```python
from build123d import *

# Parameters (mm, degrees)
CYLINDER003003_R     = 2.85
CYLINDER003003_DEPTH = 10
BOX001001004_W       = 1
BOX001001004_H       = 0.2
BOX001001004_DEPTH   = 5.1
CYLINDER002007_R     = 3.4
CYLINDER002007_DEPTH = 8.5
BOX001001005_W       = 1
BOX001001005_H       = 0.2
BOX001001005_DEPTH   = 5.1
CYLINDER004009_R     = 5
CYLINDER004009_DEPTH = 4
CHAMFER008_SIZE      = 0.5
CYLINDER001006_R     = 4
CYLINDER001006_DEPTH = 4.6
CUT003009_ROLL_ANGLE = -90


with BuildPart() as hole001:
    # Cylinder003003 → Cylinder003003 (new body)
    with BuildSketch(Plane.XY):
        Circle(CYLINDER003003_R)
    extrude(amount=CYLINDER003003_DEPTH)


with BuildPart() as contact003:
    # Box001001004 → Box001001004 (new body)
    with BuildSketch(Plane(origin=(-0.5, 2.5, -13), x_dir=(1, 0, 0), z_dir=(0, 0, 1))):
        with Locations((0.5, 0.1)):
            Rectangle(BOX001001004_W, BOX001001004_H)
    extrude(amount=BOX001001004_DEPTH)


with BuildPart() as cylinder002007:
    # Cylinder002007 → Cylinder002007 (new body)
    with BuildSketch(Plane.XY.offset(-8)):
        Circle(CYLINDER002007_R)
    extrude(amount=CYLINDER002007_DEPTH)


with BuildPart() as contact004:
    # Box001001005 → Box001001005 (new body)
    with BuildSketch(Plane(origin=(-0.5, -2.5, -13), x_dir=(1, 0, 0), z_dir=(0, 0, 1))):
        with Locations((0.5, 0.1)):
            Rectangle(BOX001001005_W, BOX001001005_H)
    extrude(amount=BOX001001005_DEPTH)


with BuildPart() as chamfer008:
    # Cylinder004009 → Cylinder004009 (new body)
    with BuildSketch(Plane.XY):
        Circle(CYLINDER004009_R)
    extrude(amount=CYLINDER004009_DEPTH)

    # Chamfer008
    chamfer008_edges = [chamfer008.edges().sort_by_distance(p)[0] for p in [
        (-5, 0, 4),
    ]]
    chamfer(chamfer008_edges, length=CHAMFER008_SIZE)


with BuildPart() as powerconnector:
    # Cylinder001006 → Cylinder001006 (new body)
    with BuildSketch(Plane.XY.offset(-4.5)):
        Circle(CYLINDER001006_R)
    extrude(amount=CYLINDER001006_DEPTH)

    # Fusion005: union contact003, Cylinder002007, contact004, Chamfer008
    add(contact003.part)
    add(cylinder002007.part)
    add(contact004.part)
    add(chamfer008.part)

    # Cut003009: cut hole001
    add(hole001.part, mode=Mode.SUBTRACT)


with BuildPart() as powerconnector_1:
    # Cut003009 roll: moved
    add(powerconnector.part.rotate(Axis((0, 0, 0), (1, 0, 0)), CUT003009_ROLL_ANGLE))


with BuildPart() as powerconnector_2:
    # Cut003009 placement: moved
    add(powerconnector_1.part.moved(Location((-0.7, 30, 39.2))))


solid = powerconnector_2.part
```
Work out the finished part from the listing and answer in its coordinate system (mm). A direction names the side the tool comes from. Give positions to 0.01 mm unless a question says otherwise; leave off trailing zeros. Write each loop counter-clockwise with the first axis right and the second up, starting at its lowest first coordinate (ties: lowest second). Pieces come first, ordered by that corner, then holes.
(1) Flat-ended cylindrical pins translate along their axes: pin 1 Ø3 at (x, z) = (-0.5, 40.5) entering from +Y; pin 2 Ø1 at (x, y) = (-4, 26) entering from +Z; pin 3 Ø0.8 at (x, y) = (-0.5, 19.5) entering from +Z; pin 4 Ø4 at (x, y) = (-1, 29) entering from +Z. Find the tip coordinate at first contact, or state that the pin passes through.
Final values:
pin 1: stops at y = 30
pin 2: stops at z = 42.06
pin 3: stops at z = 41.7
pin 4: stops at z = 44.2
(2) The part is cut by section A-A on y = 20.75. Write down the section's boundary in (x, z), plus the area to 3 significant figures.
Final values:
outline: (-1.2, 36.5) - (-0.2, 36.5) - (-0.2, 36.7) - (-1.2, 36.7) - close; (-1.2, 41.5) - (-0.2, 41.5) - (-0.2, 41.7) - (-1.2, 41.7) - close
area: 0.400 mm2
(3) The part is cut by section D-D on y = 32.5. Write down the section's boundary in (x, z).
Final values:
outline: circle Ø10 at (-0.7, 39.2); hole circle Ø5.7 at (-0.7, 39.2)
(4) The mould has two halves that part along Z. Classify faces 6 (the cylindrical face through (-1.44, 23.73, 42.52)), 7 (the flat face through (-1, 19, 36.7)), 8 (the flat face through (1, 30, 35)): pulls with the +Z half, pulls with the -Z half, needs draft (parallel to the pull), parting line crosses it, or undercut.
Final values:
face 6: parting line crosses it
face 7: undercut
face 8: needs draft
(5) Straight lines are drawn through the part: line 1 (X direction, y = 33.15, z = 39.2); line 2 (Z direction, x = -0.7, y = 31.6); line 3 (Y direction, x = 0, z = 35.75). For each, find the intervals that lie inside material, in ascending order.
Final values:
line 1: x = -5.7 to -3.55, 2.15 to 4.3
line 2: z = 34.2 to 36.35, 42.05 to 44.2
line 3: y = 25.5 to 34
(6) The part is cut by section B-B on x = -0.7. Write down the section's boundary in (y, z), plus the area to 4 significant figures.
Final values:
outline: (17, 36.5) - (22, 36.5) - (22, 35.8) - (25.5, 35.8) - (25.5, 35.2) - (30, 35.2) - (30, 34.2) - (33.5, 34.2) - (34, 34.7) - (34, 36.35) - (30, 36.35) - (30, 42.05) - (34, 42.05) - (34, 43.7) - (33.5, 44.2) - (30, 44.2) - (30, 43.2) - (25.5, 43.2) - (25.5, 42.6) - (22, 42.6) - (22, 41.7) - (17, 41.7) - (17, 41.5) - (22, 41.5) - (22, 36.7) - (17, 36.7) - close
area: 78.75 mm2
(7) The part is cut by section C-C on z = 39.2. Write down the section's boundary in (x, y), plus the area to 4 significant figures.
Final values:
outline: (-5.7, 30) - (-4.7, 30) - (-4.7, 25.5) - (-4.1, 25.5) - (-4.1, 22) - (2.7, 22) - (2.7, 25.5) - (3.3, 25.5) - (3.3, 30) - (4.3, 30) - (4.3, 33.5) - (3.8, 34) - (2.15, 34) - (2.15, 30) - (-3.55, 30) - (-3.55, 34) - (-5.2, 34) - (-5.7, 33.5) - close
area: 76.75 mm2
(8) Which of the six approach directions +Z, -Z, +X, -X, +Y, -Y give full straight-line access (tool end or side, diameter ignored) to faces 1 (the flat face through (-1, 19, 41.5)), 2 (the flat face through (-1, 19, 36.5)), 3 (the flat face through (-4, 25.5, 41)), 4 (the flat face through (-1, 19, 41.7)), 5 (the flat face through (-1, 30, 39))?
Final values:
face 1: +X, -X, -Y
face 2: -Z, +X, -X, -Y
face 3: -Y
face 4: +Z, +X, -X, -Y
face 5: +Y
